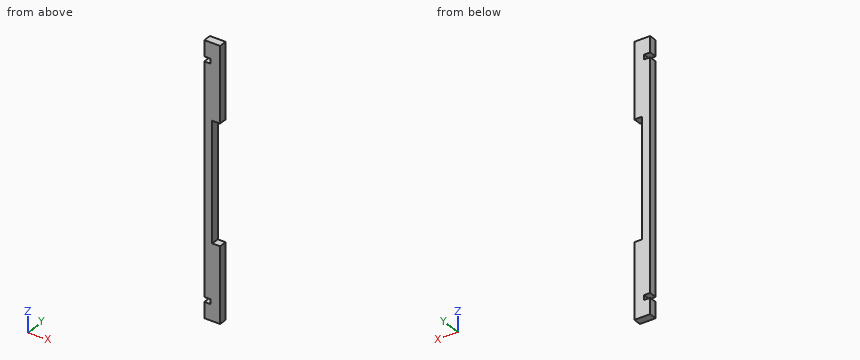
Autodesk Inventor part; units mm, degrees
ref_plane "YZ Plane" through (0, 0, 0) normal (1, 0, 0) x (0, 1, 0)
ref_plane "XZ Plane" through (0, 0, 0) normal (0, 1, 0) x (-1, 0, 0)
ref_plane "XY Plane" through (0, 0, 0) normal (0, 0, 1) x (1, 0, 0)
sketch "Sketch1" plane through (0, 0, 0) normal (0, 1, 0) x (-1, 0, 0)
  line L0 (5, 85) -> (-5, 85)
  line L1 (-5, 85) -> (-5, -85)
  line L2 (-5, -85) -> (5, -85)
  line L3 (5, -85) -> (5, 85)
  line L4 (5, 85) -> (-5, -85) construction
  line L5 (-5, 85) -> (5, -85) construction
  point P0 (0, 0)
  dimension "d0" = 170
  dimension "d1" = 10
extrude "Extrusion1" add sketch "Sketch1" along normal blind 5
sketch "Sketch2" plane through (0, 5, 0) normal (0, 1, 0) x (1, 0, 0)
  line L0 (-5, 85) -> (-5, -85)
  line L1 (-5, -75) -> (-1, -75)
  line L2 (-1, -75) -> (-1, -72)
  line L3 (-1, -72) -> (-5, -72)
  line L4 (-5, -72) -> (-5, -75)
  line L5 (-5, -85) -> (5, -85)
  line L6 (5, 0) -> (-5, 0) construction
  line L7 (-5, 75) -> (-1, 75)
  line L8 (-1, 75) -> (-1, 72)
  line L9 (-1, 72) -> (-5, 72)
  line L10 (-5, 72) -> (-5, 75)
  point P0 (0, 0)
  point P1 (-5, 75)
  point P2 (-5, 72)
  dimension "d4" = 3
  dimension "d5" = 4
  dimension "d6" = 10
extrude "Extrusion2" cut sketch "Sketch2" against normal blind 5
sketch "Sketch3" plane through (0, 5, 0) normal (0, 1, 0) x (1, 0, 0)
  line L0 (0, 37.5) -> (10, 37.5)
  line L1 (10, 37.5) -> (10, -37.5)
  line L2 (10, -37.5) -> (0, -37.5)
  line L3 (0, -37.5) -> (0, 37.5)
  line L4 (5, -85) -> (5, 85)
  line L5 (0, 37.5) -> (10, -37.5) construction
  line L6 (10, 37.5) -> (0, -37.5) construction
  point P0 (0, 0)
  point P1 (5, 0)
  point P2 (5, -37.5)
  point P3 (5, 37.5)
  dimension "d9" = 75
  dimension "d10" = 5
extrude "Extrusion3" cut sketch "Sketch3" against normal blind 10 contours L0 L4 L2 L3
properties part number "Gel top"
CAD build for the part. Positions are in the model's coordinates, mm. Round coordinates to 2 decimals unless told otherwise and drop trailing zeros. Loops run counter-clockwise (first coordinate to the right, second up) from the corner with the lowest first, then second, coordinate; pieces in that order, holes last. Notation, with made-up numbers: M 29.5,37.25 L 82.5,37.25 A16 ccw 82.5,60.25 Z; hole C -35.5,-14.5 d9. An arc over 180 degrees is marked long. Return JSON: item names as keys, results as strings. Group by question number.
(1) Saw through at C-C, the plane z = -32.5. List the corners of the cut face in (x, y), and give its area (3 significant figures).
(2) Saw through at B-B, the plane y = 2.4. List the corners of the cut face in (x, z).
(3) Saw through at A-A, the plane x = 2.25. List the corners of the cut face in (y, z).
(4) Drop flat-ended pins along their axis: P1, Ø1, axis at y = 3.5, z = 7.5, coming from the +X side; P2, Ø2.5, axis at y = 1.5, z = -73, coming from the -X side; P3, Ø1.5, axis at y = 3, z = 73, coming from the -X side. Give the stop position or say it passes through.
(5) Wall check: probe 1 along Z at (x, y) = (-1.5, 2.45); probe 2 along Z at (x, y) = (1, 0.25); probe 3 along X at (y, z) = (1.35, 15). Give the ranges that are in metal, low to high. Write a range as [from, to].
Answer list:
{
 "1": {"outline": "M -5,0 L 0,0 L 0,5 L -5,5 Z", "area": "25.0 mm2"},
 "2": {"outline": "M -5,-85 L 5,-85 L 5,-37.5 L 0,-37.5 L 0,37.5 L 5,37.5 L 5,85 L -5,85 L -5,75 L -1,75 L -1,72 L -5,72 L -5,-72 L -1,-72 L -1,-75 L -5,-75 Z"},
 "3": {"outline": "M 0,-85 L 5,-85 L 5,-37.5 L 0,-37.5 Z; M 0,37.5 L 5,37.5 L 5,85 L 0,85 Z"},
 "4": {"P1": "x = 0", "P2": "x = -5", "P3": "x = -1"},
 "5": {"probe 1": "[-85, -75], [-72, 72], [75, 85]", "probe 2": "[-85, -37.5], [37.5, 85]", "probe 3": "[-5, 0]"}
}
